Here's how the part is built. I have some questions about the finished solid (model axes, mm). Round coordinates to 2 decimals unless told otherwise and drop trailing zeros. Write each loop counter-clockwise with the first axis right and the second up, starting at its lowest first coordinate (ties: lowest second). Pieces come first, ordered by that corner, then holes. Notation, with made-up numbers: (76, 18.5) -> (118, 18.5) arc R35 ccw to (118, 56.5) -> close; hole circle Ø7 at (-39.75, -28). An arc over 180 degrees is marked (long way). Put each result on its own line as item: value. Start each with the question number.
1. For pin 1 (3 mm diameter, centred on y = -18.5, z = 8.5, fed in from +X); pin 2 (4 mm diameter, centred on x = 4, z = 7.5, fed in from -Y), each with a flat end and sliding along its axis, tell me the tip position at first contact or that it passes through.
2. Suppose I cut it at A-A (z = 3). Please give me the cut outline in (x, y).
3. Suppose I cut it at C-C (x = -13.5). Please give me the cut outline in (y, z), then the cut area to 3 significant figures.
4. I need wall thicknesses on probe 1 along Y at (x, z) = (14, 2.25); probe 2 along Y at (x, z) = (-17.5, 4.75); probe 3 along X at (y, z) = (-19, 9). Which ranges of each line are inside material? Lowest first, please. Write a range as from..to.
5. Suppose I cut it at B-B (y = -19). Please give me the cut outline in (x, z).
```python
from build123d import *

# Parameters (mm, degrees)
F0_W        = 64.6526291966
F0_H        = 71.8573257327
F1_DEPTH    = 12.192
F2_T1_DEPTH = 205.3532271255


# Not quite as in the source:
# - a fillet or chamfer that OpenCascade refuses, or shapes differently, is made with other operations: its cross-section is extruded or revolved along the edge and cut away or added


with BuildPart() as f1:
    # F0 (on Top) → F1 (new body)
    with BuildSketch(Plane.XY):
        with Locations((7.299490273, 7.4890889227)):
            Rectangle(F0_W, F0_H)
    extrude(amount=F1_DEPTH)

    # F2: fillet of radius 38.6322454251 on 2 edges, made by hand

    # F2_s2 → F2_t1 (cut)
    with BuildSketch(Plane.XY.offset(-96.5806135627)):
        with BuildLine():
            ThreePointArc((0.9935594462, -28.4395739436), (28.3106821588, -17.1244512311), (39.6258048713, 10.1926714815))
            Line((39.6258048713, 10.1926714815), (39.6258048713, -28.4395739436))
            Line((39.6258048713, -28.4395739436), (0.9935594462, -28.4395739436))
        make_face()
        with BuildLine():
            ThreePointArc((-25.0268243253, 10.1926714815), (-13.7117016128, -17.1244512311), (13.6054210998, -28.4395739436))
            Line((13.6054210998, -28.4395739436), (-25.0268243253, -28.4395739436))
            Line((-25.0268243253, -28.4395739436), (-25.0268243253, 10.1926714815))
        make_face()
    extrude(amount=F2_T1_DEPTH, mode=Mode.SUBTRACT)


solid = f1.part
```
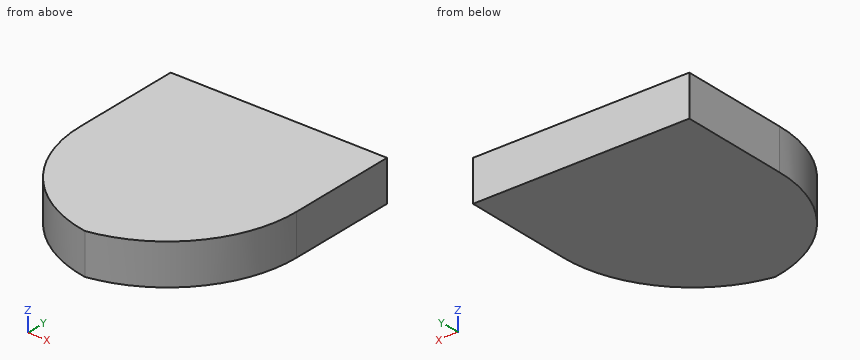
Verdict:
1. pin 1: stops at x = 28.43
1. pin 2: stops at y = -27.68
2. outline: (-25.03, 10.19) arc R38.63 ccw to (7.3, -27.92) arc R38.63 ccw to (39.63, 10.19) -> (39.63, 43.42) -> (-25.03, 43.42) -> close
3. outline: (-17.33, 0) -> (43.42, 0) -> (43.42, 12.19) -> (-17.33, 12.19) -> close
3. area: 741 mm^2
4. probe 1: y = -26.18..43.42
4. probe 2: y = -12.72..43.42
4. probe 3: x = -11.7..26.3
5. outline: (-11.7, 0) -> (26.3, 0) -> (26.3, 12.19) -> (-11.7, 12.19) -> close
